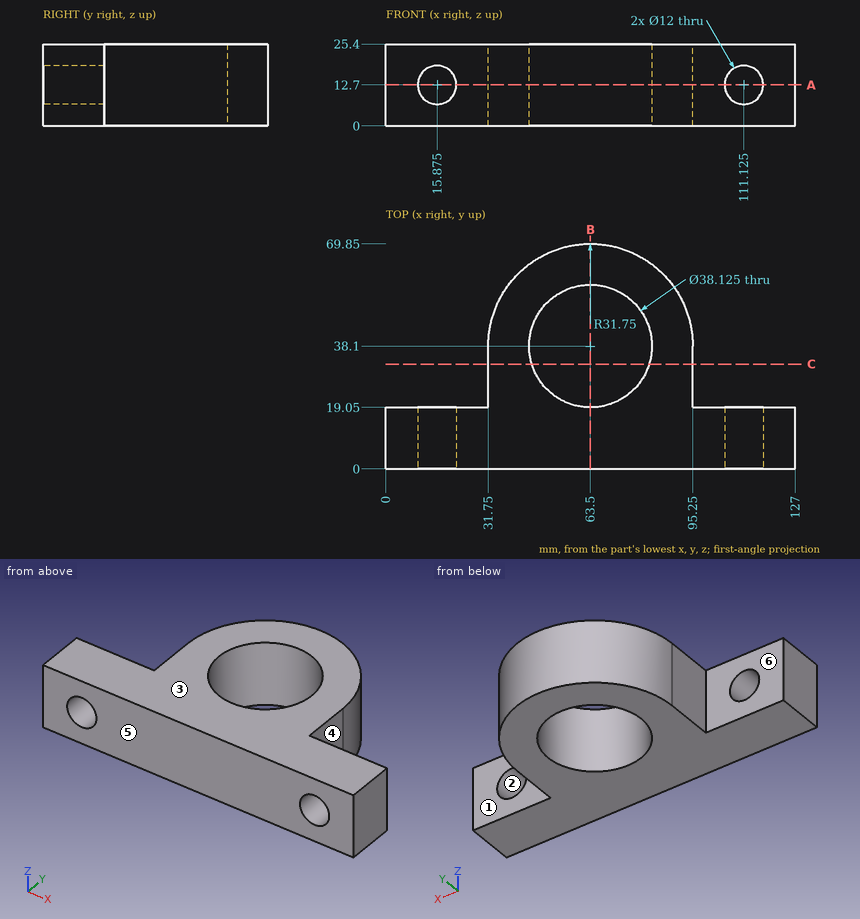
Part print with two shaded views. Sizes in mm from the minimum x, y, z corner. A direction names the side the tool comes from. Round coordinates to 2 decimals unless told otherwise and drop trailing zeros. Order: outer loops, then holes, each group sorted by start corner. A loop starts at its lowest first (then second) coordinate and runs counter-clockwise, first axis right, second up.
(1) Band-saw the part on B-B (x = 63.5). List the corners of the cut face in (y, z).
(2) Pin check, flat tips, straight feed: pin 1 (12.5 mm diameter, centred on x = 117.5, z = 15.5, fed in from +Y); pin 2 (2 mm diameter, centred on y = 47.5, z = 19, fed in from -X); pin 3 (12 mm diameter, centred on y = 8, z = 22, fed in from -X); pin 4 (8 mm diameter, centred on y = 43.5, z = 12.5, fed in from +X). Stop position of each tip, or through.
(3) Pull direction Z, two halves, no side cores. Call the marked faces 1, 2 and 3: released by +Z, released by -Z, zero draft, split by the parting line, or undercut.
(4) 3-axis set-ups, long thin cutter, end or side, ignore diameter. For the marked faces 4, 5 and 6: which of +Z, -Z, +X, -X, +Y, -Y reach the whole face in a straight line?
(5) Band-saw the part on C-C (y = 32.5). List the corners of the cut face in (x, z).
(6) Band-saw the part on A-A (z = 12.7). Give the number of separate pieces and of enclosed holes in the cut face, then the cut area to 3 significant figures.
(7) Drill centre lines: line 1 (X direction, y = 12, z = 11.5); line 2 (Y direction, x = 55.5, z = 1.5) (1 decimal); line 3 (Y direction, x = 57.5, z = 14.5) (1 decimal). Where is each one in solid material? Low to high.
Verdict:
1. outline: (0, 0) - (19.04, 0) - (19.04, 25.4) - (0, 25.4) - close; (57.16, 0) - (69.85, 0) - (69.85, 25.4) - (57.16, 25.4) - close
2. pin 1: stops at y = 19.05
2. pin 2: stops at x = 32.88
2. pin 3: stops at x = 0
2. pin 4: stops at x = 95.22
3. face 1: zero draft
3. face 2: undercut
3. face 3: released by +Z
4. face 4: +Z, -Z, +X, +Y
4. face 5: +Z, -Z, +X, -X, -Y
4. face 6: +Z, -Z, -X, +Y
5. outline: (31.75, 0) - (45.28, 0) - (45.28, 25.4) - (31.75, 25.4) - close; (81.72, 0) - (95.25, 0) - (95.25, 25.4) - (81.72, 25.4) - close
6. separate pieces: 3
6. enclosed holes: 1
6. area: 3,610 mm2
7. line 1: x = 0 to 10, 21.75 to 105.25, 117 to 127
7. line 2: y = 0 to 20.8, 55.4 to 68.8
7. line 3: y = 0 to 20, 56.2 to 69.3
